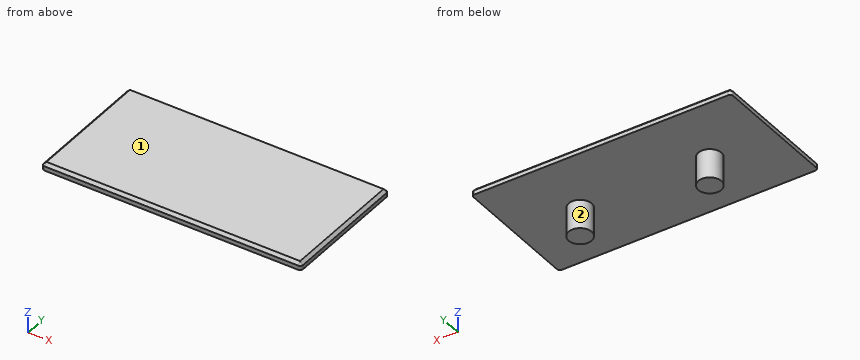
```python
from build123d import *

# Parameters (mm, degrees)
SKETCH1_W           = 90
SKETCH1_H           = 45
BOSS_EXTRUDE1_DEPTH = 2.5
FILLET1_R           = 1
CHAMFER1_SIZE       = 1
SKETCH2_R           = 4
BOSS_EXTRUDE2_DEPTH = 10


with BuildPart() as part:
    # Sketch1 → Boss-Extrude1 (new body)
    with BuildSketch(Plane.XY):
        Rectangle(SKETCH1_W, SKETCH1_H)
    extrude(amount=BOSS_EXTRUDE1_DEPTH)

    # Fillet1
    fillet1_edges = [part.edges().sort_by_distance(p)[0] for p in [
        (45, -22.5, 1.25),
        (-45, -22.5, 1.25),
        (-45, 22.5, 1.25),
        (45, 22.5, 1.25),
    ]]
    fillet(fillet1_edges, radius=FILLET1_R)

    # Chamfer1
    chamfer1_edges = [part.edges().sort_by_distance(p)[0] for p in [
        (0, -22.5, 2.5),
        (-45, 0, 2.5),
        (45, 0, 2.5),
        (0, 22.5, 2.5),
        (44.707106781, -22.207106781, 2.5),
        (44.707106781, 22.207106781, 2.5),
        (-44.707106781, 22.207106781, 2.5),
        (-44.707106781, -22.207106781, 2.5),
    ]]
    chamfer(chamfer1_edges, length=CHAMFER1_SIZE)

    # Sketch2 → Boss-Extrude2 (add)
    with BuildSketch(Plane(origin=(0, 0, 0), x_dir=(-1, 0, 0), z_dir=(0, 0, -1))):
        with Locations((-22.5, 0)):
            Circle(SKETCH2_R)
        with Locations((22.5, 0)):
            Circle(SKETCH2_R)
    extrude(amount=BOSS_EXTRUDE2_DEPTH)


solid = part.part
```
The listing builds one solid part. Answer for the finished solid, in the listing's coordinates (mm). Face numbers are marked on the shaded views. A direction names the side the tool comes from. Coordinates: 2 decimals unless noted, no trailing zeros. Write each loop counter-clockwise with the first axis right and the second up, starting at its lowest first coordinate (ties: lowest second). Pieces come first, ordered by that corner, then holes.
Q1. Find the intervals of material crossed by line 1 along Y through (x, z) = (-22.5, -7.5); line 2 along Z through (x, y) = (-37, 1); line 3 along X through (y, z) = (-2, -7), in increasing order.
Returned:
line 1: y = -4 to 4
line 2: z = 0 to 2.5
line 3: x = -25.96 to -19.04, 19.04 to 25.96
Q2. Section C-C, the plane z = -2 is taken. Write down the section's boundary in (x, y).
Returned:
outline: circle Ø8 at (-22.5, 0); circle Ø8 at (22.5, 0)
Q3. Section B-B, the plane y = 0 is taken. Write down the section's boundary in (x, z).
Returned:
outline: (-45, 0) - (-26.5, 0) - (-26.5, -10) - (-18.5, -10) - (-18.5, 0) - (18.5, 0) - (18.5, -10) - (26.5, -10) - (26.5, 0) - (45, 0) - (45, 1.5) - (44, 2.5) - (-44, 2.5) - (-45, 1.5) - close
Q4. Section D-D, the plane x = 22.5 is taken. Write down the section's boundary in (y, z), then the cut area to 4 significant figures.
Returned:
outline: (-22.5, 0) - (-4, 0) - (-4, -10) - (4, -10) - (4, 0) - (22.5, 0) - (22.5, 1.5) - (21.5, 2.5) - (-21.5, 2.5) - (-22.5, 1.5) - close
area: 191.5 mm2
Q5. Given P1, Ø1, axis at x = -24, y = 5, coming from the -Z side; P2, Ø6, axis at x = -16, z = -3.5, coming from the -Y side; P3, Ø6, axis at x = -11.5, z = -4.5, coming from the +Y side; P4, Ø3, axis at x = 24, z = -3.5, coming from the +Y side, each flat-ended and moving along its own axis, determine where each tip first touches the part or whether it passes through.
Returned:
P1: stops at z = 0
P2: stops at y = -1.94
P3: passes through
P4: stops at y = 4
Q6. Which of the six approach directions +Z, -Z, +X, -X, +Y, -Y give full straight-line access (tool end or side, diameter ignored) to the marked faces 1 and 2?
Returned:
face 1: +Z, +X, -X, +Y, -Y
face 2: -Z
Q7. Section A-A, the plane x = 12 is taken. Write down the section's boundary in (y, z), then the cut area to 4 significant figures.
Returned:
outline: (-22.5, 0) - (22.5, 0) - (22.5, 1.5) - (21.5, 2.5) - (-21.5, 2.5) - (-22.5, 1.5) - close
area: 111.5 mm2
